```python
from build123d import *

# Parameters (mm, degrees)
SKETCH1_W           = 54
SKETCH1_H           = 32
BOSS_EXTRUDE1_DEPTH = 2
SKETCH2_W           = 54
SKETCH2_H           = 32
SKETCH2_W_2         = 50
SKETCH2_H_2         = 28
BOSS_EXTRUDE2_DEPTH = 2
SKETCH3_W           = 2
SKETCH3_H           = 10
CUT_EXTRUDE1_DEPTH  = 4
SKETCH4_W           = 7.76
SKETCH4_H           = 23.32
BOSS_EXTRUDE3_DEPTH = 7.38
SKETCH5_R           = 2.4
CUT_EXTRUDE2_DEPTH  = 7.79
SKETCH6_R           = 3.1
CUT_EXTRUDE3_DEPTH  = 0.8
CUT_EXTRUDE4_START  = -0.8
SKETCH7_R           = 3.1
CUT_EXTRUDE4_DEPTH  = 0.8
FILLET1_R           = 3.69


with BuildPart() as part:
    # Sketch1 → Boss-Extrude1 (new body)
    with BuildSketch(Plane(origin=(0, 0, 0), x_dir=(1, 0, 0), z_dir=(0, 1, 0))):
        with Locations((27, 16)):
            Rectangle(SKETCH1_W, SKETCH1_H)
    extrude(amount=BOSS_EXTRUDE1_DEPTH)

    # Sketch2 → Boss-Extrude2 (add)
    with BuildSketch(Plane(origin=(0, 2, 0), x_dir=(1, 0, 0), z_dir=(0, 1, 0))):
        with Locations((27, 16)):
            Rectangle(SKETCH2_W, SKETCH2_H)
        with Locations((27, 16)):
            Rectangle(SKETCH2_W_2, SKETCH2_H_2, mode=Mode.SUBTRACT)
    extrude(amount=BOSS_EXTRUDE2_DEPTH)

    # Sketch3 → Cut-Extrude1 (cut)
    with BuildSketch(Plane(origin=(0, 4, 0), x_dir=(1, 0, 0), z_dir=(0, 1, 0))):
        with Locations((1, 16)):
            Rectangle(SKETCH3_W, SKETCH3_H)
        with Locations((53, 16)):
            Rectangle(SKETCH3_W, SKETCH3_H)
    extrude(amount=-CUT_EXTRUDE1_DEPTH, mode=Mode.SUBTRACT)

    # Sketch4 → Boss-Extrude3 (add)
    with BuildSketch(Plane.XZ):
        with Locations((27, -11.66)):
            Rectangle(SKETCH4_W, SKETCH4_H)
    extrude(amount=BOSS_EXTRUDE3_DEPTH)

    # Sketch5 → Cut-Extrude2 (cut)
    with BuildSketch(Plane(origin=(30.88, 0, 0), x_dir=(0, 0, -1), z_dir=(1, 0, 0))):
        with Locations((3.69, -3.69)):
            Circle(SKETCH5_R)
        with Locations((11.66, -3.69)):
            Circle(SKETCH5_R)
        with Locations((19.63, -3.69)):
            Circle(SKETCH5_R)
    extrude(amount=-CUT_EXTRUDE2_DEPTH, mode=Mode.SUBTRACT)

    # Sketch6 → Cut-Extrude3 (cut)
    with BuildSketch(Plane.ZY.offset(-23.12)):
        with Locations((-11.66, -3.69)):
            Circle(SKETCH6_R)
        with Locations((-3.69, -3.69)):
            Circle(SKETCH6_R)
        with Locations((-19.63, -3.69)):
            Circle(SKETCH6_R)
    extrude(amount=-CUT_EXTRUDE3_DEPTH, mode=Mode.SUBTRACT)

    # Sketch7 → Cut-Extrude4 (cut)
    with BuildSketch(Plane(origin=(30.88, 0, 0), x_dir=(0, 0, -1), z_dir=(1, 0, 0)).offset(CUT_EXTRUDE4_START)):
        with Locations(Location((3.69, -3.69, 0), (0, 0, 180))):
            Circle(SKETCH7_R)
        with Locations(Location((11.66, -3.69, 0), (0, 0, 180))):
            Circle(SKETCH7_R)
        with Locations(Location((19.63, -3.69, 0), (0, 0, 180))):
            Circle(SKETCH7_R)
    extrude(amount=CUT_EXTRUDE4_DEPTH, mode=Mode.SUBTRACT)

    # Fillet1
    fillet1_edges = [part.edges().sort_by_distance(p)[0] for p in [
        (27, -7.38, -23.32),
        (27, -7.38, 0),
    ]]
    fillet(fillet1_edges, radius=FILLET1_R)


solid = part.part
```
Source: CAD feature listing. Evaluate the final solid. Frame: model axes, mm. A direction names the side the tool comes from. Round coordinates to 2 decimals unless told otherwise and drop trailing zeros. Write each loop counter-clockwise with the first axis right and the second up, starting at its lowest first coordinate (ties: lowest second). Pieces come first, ordered by that corner, then holes. Notation, with made-up numbers: M -15,25.5 L 0,25.5 A22 cw 0,60.5 Z; hole C -19,24.25 d7. An arc over 180 degrees is marked long. Use CSV: the item, a comma, the result in double quotes. Start each with the question number.
Q1. Pull-direction query (Y, two-part tool) for faces 1 (the face through (30.474, -4.621, -16.673)), 2 (the face through (27, 2, -16)), 3 (the face through (2, 3, -6)); classes: +Y half, -Y half, draft (parallel to the pull), parting line (faces both ways), or undercut.
Q2. Line query: line 1 (X direction, y = 3.25, z = -27); line 2 (Y direction, x = 26.5, z = -19.63); line 3 (Z direction, x = 46, y = 3.25). Output: solid intervals per line, ascending. Write a range as from..to.
Q3. Cut plane C-C on x = 27. Output: boundary loops of the cut face in (y, z).
Q4. Access query for faces 4 (the face through (27, 3, -30)), 5 (the face through (23.5, -5.6, -14.1)), 6 (the face through (30.08, -1, -3)), 7 (the face through (1, 2, -21)). Directions: +Z, -Z, +X, -X, +Y, -Y. A direction counts if a zero-diameter tool reaches every point of the face in a straight line with its end or side. Return the directions, or none.
Q5. First-contact query: P1, Ø3, axis at x = 16, z = -7, coming from the -Y side; P2, Ø1.6, axis at y = 1.5, z = -15, coming from the -X side; P3, Ø1.1, axis at x = 29, y = -1, coming from the -Z side; P4, Ø3.5, axis at y = -3.69, z = -19.63, coming from the +X side. Flat tips, straight axial feed; report the tip coordinate or a pass-through.
Q6. Cut plane D-D on x = 40. Output: boundary loops of the cut face in (y, z), plus the area to 3 significant figures.
Q7. Cut plane A-A on z = -11.66. Output: boundary loops of the cut face in (x, y).
Q8. Cut plane B-B on y = 2.75. Output: boundary loops of the cut face in (x, z), plus the area to 3 significant figures.
Results found:
1,face 1,"undercut"
1,face 2,"+Y half"
1,face 3,"draft"
2,line 1,"0..2, 52..54"
2,line 2,"-7.38..-6.09, -1.29..2"
2,line 3,"-32..-30, -2..0"
3,outline,"M -7.38,-19.63 A3.69 ccw -3.69,-23.32 L 0,-23.32 L 0,-32 L 4,-32 L 4,-30 L 2,-30 L 2,-2 L 4,-2 L 4,0 L -3.69,0 A3.69 ccw -7.38,-3.69 Z; hole C -3.69,-19.63 d4.8; hole C -3.69,-11.66 d4.8; hole C -3.69,-3.69 d4.8"
4,face 4,"+Y"
4,face 5,"-X"
4,face 6,"+X"
4,face 7,"-X, +Y, -Y"
5,P1,"y = 0"
5,P2,"x = 2"
5,P3,"z = -23.32"
5,P4,"through"
6,outline,"M 0,-32 L 4,-32 L 4,-30 L 2,-30 L 2,-2 L 4,-2 L 4,0 L 0,0 Z"
6,area,"72.0 mm^2"
7,outline,"M 2,0 L 23.12,0 L 23.12,-0.59 L 23.92,-0.59 L 23.92,-1.29 L 30.08,-1.29 L 30.08,-0.59 L 30.88,-0.59 L 30.88,0 L 52,0 L 52,2 L 2,2 Z; M 23.12,-7.38 L 30.88,-7.38 L 30.88,-6.79 L 30.08,-6.79 L 30.08,-6.09 L 23.92,-6.09 L 23.92,-6.79 L 23.12,-6.79 Z"
8,outline,"M 0,-32 L 54,-32 L 54,-21 L 52,-21 L 52,-30 L 2,-30 L 2,-21 L 0,-21 Z; M 0,-11 L 2,-11 L 2,-2 L 52,-2 L 52,-11 L 54,-11 L 54,0 L 0,0 Z"
8,area,"288 mm^2"
